Geometry check sheet. Reference: the model listing, model coordinates, mm. Give positions to 0.01 mm unless a question says otherwise; leave off trailing zeros. Order: outer loops, then holes, each group sorted by start corner. A loop starts at its lowest first (then second) coordinate and runs counter-clockwise, first axis right, second up.
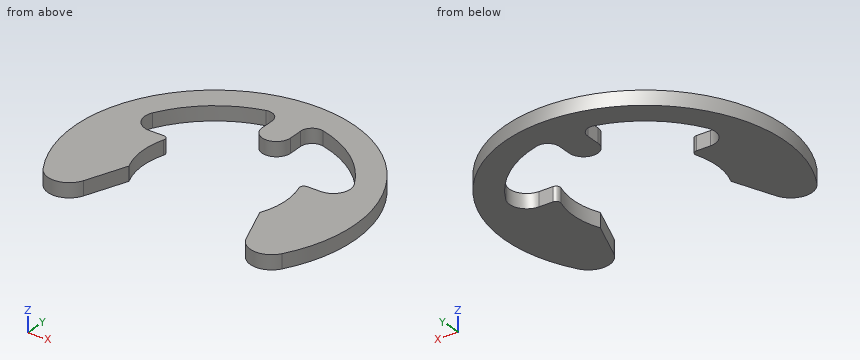
Autodesk Inventor part; units mm, degrees
ref_plane "Work Plane1" through (0, -7.9764, 0) normal (-1, 0, 0) x (0, 0, 1)
ref_plane "YZ Plane" through (0, 0, 0) normal (1, 0, 0) x (0, 1, 0)
ref_plane "XZ Plane" through (0, 0, 0) normal (0, 1, 0) x (-1, 0, 0)
sketch "Sketch1" plane through (0, 0, 0) normal (0, 0, 1) x (1, 0, 0)
  circle A0 centre (0, -7.9764) radius 8 construction
  line L0 (-1.5, 0.0236) -> (0, 0.0236) construction
  line L1 (-3.206, 0) -> (3.4858, 0)
  line L2 (-6.8739, -10.9764) -> (6.8739, -10.9764) construction
  arc A1 (-7.1037, -5.5707) -> (-6.8739, -10.9764) centre (0, -7.9764) ccw
  line L3 (0, 1.949) -> (0, -3.4788)
  arc A2 (-1.5, 1.0236) -> (1.5, 1.0236) centre (0, 1.0236) ccw
  arc A3 (12.5579, -15.6176) -> (-12.5579, -15.6176) centre (0, -7.9764) ccw
  line L4 (-9, -4.9764) -> (-7.5299, -4.9764)
  line L5 (-1.5, 1.0236) -> (-1.5, 2.4807)
  arc A4 (-3, 3.6426) -> (-10.5882, -2.3293) centre (0, -7.9764) ccw
  arc A5 (-1.5, 2.4807) -> (-3, 3.6426) centre (-2.7, 2.4807) ccw
  arc A6 (-10.5882, -2.3293) -> (-9, -4.9764) centre (-9, -3.1764) ccw
  arc A7 (-7.1037, -5.5707) -> (-7.5299, -4.9764) centre (-7.5299, -5.4264) ccw
  line L6 (0, 6.7236) -> (2.5298, 6.7236) construction
  line L7 (-6.8739, -10.9764) -> (-8.5384, -15.2625)
  arc A8 (-12.5579, -15.6176) -> (-8.5384, -15.2625) centre (-10.6358, -14.448) ccw
  line L8 (0, -0.4764) -> (-1.2778, -0.4764) construction
  line L9 (6.8739, -10.9764) -> (8.5384, -15.2625)
  arc A9 (8.5384, -15.2625) -> (12.5579, -15.6176) centre (10.6358, -14.448) ccw
  arc A10 (6.8739, -10.9764) -> (7.1037, -5.5707) centre (0, -7.9764) ccw
  line L10 (9, -4.9764) -> (7.5299, -4.9764)
  line L11 (1.5, 1.0236) -> (1.5, 2.4807)
  arc A11 (10.5882, -2.3293) -> (3, 3.6426) centre (0, -7.9764) ccw
  arc A12 (3, 3.6426) -> (1.5, 2.4807) centre (2.7, 2.4807) ccw
  arc A13 (9, -4.9764) -> (10.5882, -2.3293) centre (9, -3.1764) ccw
  arc A14 (7.5299, -4.9764) -> (7.1037, -5.5707) centre (7.5299, -5.4264) ccw
  point P0 (1.5, 0.0236)
  dimension "d0" = 16
  dimension "d3" = 3
  dimension "d4" = 1.5
  dimension "d5" = 29.4
  dimension "d8" = 12
  dimension "d9" = 3
  dimension "d10" = 1.2
  dimension "d11" = 1.8
  dimension "d12" = 0.45
  dimension "d13" = 2.25
  dimension "d14" = 7.5
  dimension "d15" = 7.5
extrude "Body" add sketch "Sketch1" along normal blind 1.5
ref_plane "Work Plane1" through (0, -7.9764, 0) normal (-1, 0, 0) x (0, 0, 1)
equation "\"d0\" = WD"
equation "\"d3\" = 0.2 * ND"
equation "\"d4\" = 0.1 * ND"
equation "\"d5\" = SD2"
equation "\"d8\" = 0.8 * ND"
equation "\"d9\" = 0.2 * ND"
equation "\"d10\" = 0.08 * ND"
equation "\"d11\" = 0.12 * ND"
equation "\"d12\" = 0.03 * ND"
equation "\"d13\" = 0.15 * ND"
equation "\"d14\" = 0.5 * ND"
equation "\"d15\" = 0.5 * ND"
equation "\"d16\" = SD"
equation "\"ND\" = 15"
equation "\"SD\" = 1.5"
equation "\"WD\" = 16"
equation "\"d1\" = 1.6 * ND"
equation "\"d2\" = ND"
equation "\"SD2\" = 29.4"
equation "\"d6\" = ND"
equation "\"d7\" = 0.15 * ND"
equation "\"WDMIN\" = 13"
equation "\"SNB\" = 1.55"
equation "\"WDMAX\" = 18"
equation "\"BUBRMI\" = 2.5"
properties part number "DIN 6799 - 15" material "Steel, Mild"
Q1. Cross-section at A-A, the plane x = 10. Record the boundary of the cut face in (y, z), and give its area (3 significant figures).
Q2. Cross-section at C-C, the plane y = 3.25. Record the boundary of the cut face in (x, z).
Q3. Thickness scan on L1, parallel to Y at x = 9.75, z = 0.8; L2, parallel to Y at x = 9, z = 0.4; L3, parallel to X at y = 0.5, z = 0.25. Record the ranges inside material, lowest first.
Q4. Cross-section at B-B, the plane y = -8. Record the boundary of the cut face in (x, z), and give its area (3 significant figures).
Q5. Cross-section at D-D, the plane z = 0.8. Record the boundary of the cut face in (x, y).
Q6. Gauge pin test, flat end, axial feed: P1, Ø0.7, axis at x = -8.5, z = 0.5, coming from the +Y side. Record the tip position at first contact, or that the pin passes through.
Answers follow:
1. outline: (-16.61, 0) - (-4.67, 0) - (-4.67, 1.5) - (-16.61, 1.5) - close; (-1.34, 0) - (2.8, 0) - (2.8, 1.5) - (-1.34, 1.5) - close
1. area: 24.1 mm2
2. outline: (-9.49, 0) - (-4.24, 0) - (-4.24, 1.5) - (-9.49, 1.5) - close; (-1.78, 0) - (1.78, 0) - (1.78, 1.5) - (-1.78, 1.5) - close; (4.24, 0) - (9.49, 0) - (9.49, 1.5) - (4.24, 1.5) - close
3. L1: y = -16.52 to -4.81, -0.98 to 3.02
3. L2: y = -15.99 to -4.98, -0.04 to 3.65
3. L3: x = -12.01 to -8.49, -1.41 to 1.41, 8.49 to 12.01
4. outline: (-14.7, 0) - (-7.5, 0) - (-7.5, 1.5) - (-14.7, 1.5) - close; (7.5, 0) - (14.7, 0) - (14.7, 1.5) - (7.5, 1.5) - close
4. area: 21.6 mm2
5. outline: (-12.56, -15.62) arc R2.25 ccw to (-8.54, -15.26) - (-6.87, -10.98) arc R7.5 cw to (-7.1, -5.57) arc R0.45 ccw to (-7.53, -4.98) - (-9, -4.98) arc R1.8 cw to (-10.59, -2.33) arc R12 cw to (-3, 3.64) arc R1.2 cw to (-1.5, 2.48) - (-1.5, 1.02) arc R1.5 ccw to (1.5, 1.02) - (1.5, 2.48) arc R1.2 cw to (3, 3.64) arc R12 cw to (10.59, -2.33) arc R1.8 cw to (9, -4.98) - (7.53, -4.98) arc R0.45 ccw to (7.1, -5.57) arc R7.5 cw to (6.87, -10.98) - (8.54, -15.26) arc R2.25 ccw to (12.56, -15.62) arc R14.7 ccw (long way) to start
6. P1: stops at y = 4.26
